```python
from build123d import *

# Parameters (mm, degrees)
F0_R     = 3
F1_DEPTH = 11
F2_R     = 4
F3_DEPTH = 1.3
F4_SIZE2 = 1.1
F4_SIZE  = 3
F5_R     = 2


with BuildPart() as f1:
    # F0 (on Top) → F1 (new body)
    with BuildSketch(Plane.XY):
        Circle(F0_R)
    extrude(amount=F1_DEPTH)

    # F2 (on face) → F3 (join)
    with BuildSketch(Plane.XY.offset(11)):
        Circle(F2_R)
    extrude(amount=F3_DEPTH)

    # F4
    f4_edges = [f1.edges().sort_by_distance(p)[0] for p in [
        (-4, 0, 12.3),
    ]]
    f4_side = f1.faces().sort_by_distance((0, 0, 12.3))[0]
    chamfer(f4_edges, length=F4_SIZE, length2=F4_SIZE2, reference=f4_side)

    # F5
    f5_edges = [f1.edges().sort_by_distance(p)[0] for p in [
        (-1, 0, 12.3),
    ]]
    fillet(f5_edges, radius=F5_R)


solid = f1.part
```
Work out the finished part from the listing and answer in its coordinate system (mm). A direction names the side the tool comes from. Coordinates: 2 decimals unless noted, no trailing zeros. Loops run counter-clockwise (first coordinate to the right, second up) from the corner with the lowest first, then second, coordinate; pieces in that order, holes last.
1) Flat-ended cylindrical pins translate along their axes: pin 1 (1 mm diameter, centred on y = 0, z = 7.5, fed in from -X); pin 2 (3 mm diameter, centred on x = -2.5, z = 10.5, fed in from -Y); pin 3 (1.5 mm diameter, centred on x = 1, z = 6.5, fed in from -Y). Find the tip coordinate at first contact, or state that the pin passes through.
Results:
pin 1: stops at x = -3
pin 2: stops at y = -3.85
pin 3: stops at y = -2.99
2) For faces 1 (the flat face through (1, 3, 11)), 2 (the flat face through (0, 0, 0)), determine the directions among +Z, -Z, +X, -X, +Y, -Y from which every point of the face is accessible in a straight line to the end or side of a thin tool.
Results:
face 1: -Z
face 2: -Z, +X, -X, +Y, -Y
3) Consider probe 1 along Y at (x, z) = (0, 10.5); probe 2 along X at (y, z) = (-0.25, 10); probe 3 along X at (y, z) = (-2, 10). Determine where each line is inside the solid, lowest interval first.
Results:
probe 1: y = -3 to 3
probe 2: x = -2.99 to 2.99
probe 3: x = -2.24 to 2.24
4) Section A-A (z = 1.5) is taken. Give the vertices of the cut face in (x, y).
Results:
outline: circle Ø6 at (0, 0)
